```python
from build123d import *
from build123d.topology import SkipClean

# Parameters (mm, degrees)
ESBO_O1_R                  = 0.75
ESBO_O1_R_2                = 1.5
RESSALTO_EXTRUS_O1_DEPTH   = 2
ESBO_O3_R                  = 3.75
ESBO_O3_R_2                = 2.5
RESSALTO_EXTRUS_O2_DEPTH   = 1.5
RESSALTO_EXTRUS_O3_DEPTH   = 1.5
CORTE_EXTRUS_O1_DEPTH      = 19.95718861
CORTE_EXTRUS_O1_DEPTH_BACK = 19.95718861
RESSALTO_EXTRUS_O4_START   = 2
ESBO_O7_R                  = 3.75
ESBO_O7_R_2                = 1.5
RESSALTO_EXTRUS_O4_DEPTH   = 2
ESBO_O8_R                  = 2.5
CORTE_EXTRUS_O2_DEPTH      = 3
RESSALTO_EXTRUS_O5_START   = 3
RESSALTO_EXTRUS_O5_DEPTH   = 3


with BuildPart() as part:
    # Esboço1 → Ressalto-extrusão1 (new body)
    with BuildSketch(Plane(origin=(0, 0, 0), x_dir=(1, 0, 0), z_dir=(0, 1, 0))):
        with BuildLine():
            Line((0.297619048, 3.738171064), (15.948412698, 2.492114043))
            ThreePointArc((15.948412698, 2.492114043), (18.25, 0), (15.948412698, -2.492114043))
            Line((15.948412698, -2.492114043), (0.297619048, -3.738171064))
            ThreePointArc((0.297619048, -3.738171064), (-3.75, 0), (0.297619048, 3.738171064))
        make_face()
        with Locations(Location((15.75, 0, 0), (0, 0, 270))):
            Circle(ESBO_O1_R, mode=Mode.SUBTRACT)
        with Locations(Location((0, 0, 0), (0, 0, 270))):
            Circle(ESBO_O1_R_2, mode=Mode.SUBTRACT)
        with Locations(Location((13.25, 0, 0), (0, 0, 270))):
            Circle(ESBO_O1_R, mode=Mode.SUBTRACT)
        with Locations(Location((10.75, 0, 0), (0, 0, 270))):
            Circle(ESBO_O1_R, mode=Mode.SUBTRACT)
        with Locations(Location((8.25, 0, 0), (0, 0, 270))):
            Circle(ESBO_O1_R, mode=Mode.SUBTRACT)
        with Locations(Location((5.75, 0, 0), (0, 0, 270))):
            Circle(ESBO_O1_R, mode=Mode.SUBTRACT)
    extrude(amount=RESSALTO_EXTRUS_O1_DEPTH)

    # Esboço3 → Ressalto-extrusão2 (add)
    with SkipClean():  # the faces are left unmerged after this step: merging them gives an invalid solid
        with BuildSketch(Plane(origin=(0, 2, 0), x_dir=(1, 0, 0), z_dir=(0, 1, 0))):
            with Locations(Location((0, 0, 0), (0, 0, 85.447928579))):
                Circle(ESBO_O3_R)
            with Locations(Location((0, 0, 0), (0, 0, 270))):
                Circle(ESBO_O3_R_2, mode=Mode.SUBTRACT)
        extrude(amount=RESSALTO_EXTRUS_O2_DEPTH)

    # Esboço5 → Ressalto-extrusão3 (add)
    with SkipClean():  # the faces are left unmerged after this step: merging them gives an invalid solid
        with BuildSketch(Plane(origin=(0, 2, 0), x_dir=(1, 0, 0), z_dir=(0, 1, 0))):
            with BuildLine():
                Line((5, 2.360620906), (5, 3.36378527))
                Line((5, 3.36378527), (0.297619048, 3.738171064))
                ThreePointArc((0.297619048, 3.738171064), (1.642055332, 3.37137276), (2.759721595, 2.538983403))
                Line((2.759721595, 2.538983403), (5, 2.360620906))
            make_face()
            with BuildLine():
                Line((5, 0.5), (3.716517187, 0.5))
                ThreePointArc((3.716517187, 0.5), (3.75, 0), (3.716517187, -0.5))
                Line((3.716517187, -0.5), (5, -0.5))
                Line((5, -0.5), (5, 0.5))
            make_face()
            with BuildLine():
                Line((5, -2.360620906), (2.759721595, -2.538983403))
                ThreePointArc((2.759721595, -2.538983403), (1.642055332, -3.37137276), (0.297619048, -3.738171064))
                Line((0.297619048, -3.738171064), (5, -3.36378527))
                Line((5, -3.36378527), (5, -2.360620906))
            make_face()
        extrude(amount=RESSALTO_EXTRUS_O3_DEPTH)

    # Esboço6 → Corte-extrusão1 (cut, two sides: drawn at the far end of the back side and taken through both)
    with SkipClean():  # the faces are left unmerged after this step: merging them gives an invalid solid
        with BuildSketch(Plane.XY.offset(-CORTE_EXTRUS_O1_DEPTH_BACK)):
            Polygon((3.716517187, 3.5), (5, 2), (5, 3.5), align=None)
        extrude(amount=CORTE_EXTRUS_O1_DEPTH + CORTE_EXTRUS_O1_DEPTH_BACK, mode=Mode.SUBTRACT)

    # Esboço7 → Ressalto-extrusão4 (add)
    with SkipClean():  # the faces are left unmerged after this step: merging them gives an invalid solid
        with BuildSketch(Plane.XZ.offset(RESSALTO_EXTRUS_O4_START)):
            with Locations(Location((0, 0, 0), (0, 0, 270))):
                Circle(ESBO_O7_R)
            with Locations(Location((0, 0, 0), (0, 0, 270))):
                Circle(ESBO_O7_R_2, mode=Mode.SUBTRACT)
        extrude(amount=-RESSALTO_EXTRUS_O4_DEPTH)

    # Esboço8 → Corte-extrusão2 (cut)
    with SkipClean():  # the faces are left unmerged after this step: merging them gives an invalid solid
        with BuildSketch(Plane.XZ.offset(2)):
            with Locations(Location((0, 0, 0), (0, 0, 90))):
                Circle(ESBO_O8_R)
        extrude(amount=-CORTE_EXTRUS_O2_DEPTH, mode=Mode.SUBTRACT)

    # Esboço9 → Ressalto-extrusão5 (add)
    with SkipClean():  # the faces are left unmerged after this step: merging them gives an invalid solid
        with BuildSketch(Plane.XZ.offset(-1).offset(RESSALTO_EXTRUS_O5_START)):
            with BuildLine():
                Line((-0.3, 2.481934729), (0, 2.181934729))
                Line((0, 2.181934729), (0.3, 2.481934729))
                ThreePointArc((0.3, 2.481934729), (0, 2.5), (-0.3, 2.481934729))
            make_face()
            with BuildLine():
                Line((0.444891262, 2.460095885), (0.643136552, 2.084997491))
                Line((0.643136552, 2.084997491), (1.018234946, 2.283242781))
                ThreePointArc((1.018234946, 2.283242781), (0.736887936, 2.388932014), (0.444891262, 2.460095885))
            make_face()
            with BuildLine():
                Line((1.150251983, 2.219666726), (1.229127598, 1.802799076))
                Line((1.229127598, 1.802799076), (1.645995248, 1.881674691))
                ThreePointArc((1.645995248, 1.881674691), (1.408300145, 2.065596936), (1.150251983, 2.219666726))
            make_face()
            with BuildLine():
                Line((1.753407768, 1.782010437), (1.705905264, 1.360414052))
                Line((1.705905264, 1.360414052), (2.127501649, 1.312911548))
                ThreePointArc((2.127501649, 1.312911548), (1.954578706, 1.558724505), (1.753407768, 1.782010437))
            make_face()
            with BuildLine():
                Line((2.200765578, 1.186014701), (2.031105761, 0.797150269))
                Line((2.031105761, 0.797150269), (2.419970193, 0.627490452))
                ThreePointArc((2.419970193, 0.627490452), (2.327184372, 0.913352561), (2.200765578, 1.186014701))
            make_face()
            with BuildLine():
                Line((2.452575708, 0.484636354), (2.175833597, 0.163056187))
                Line((2.175833597, 0.163056187), (2.497413764, -0.113685925))
                ThreePointArc((2.497413764, -0.113685925), (2.493009493, 0.186825234), (2.452575708, 0.484636354))
            make_face()
            with BuildLine():
                Line((2.486463724, -0.25980406), (2.12722907, -0.485526154))
                Line((2.12722907, -0.485526154), (2.352951164, -0.844760808))
                ThreePointArc((2.352951164, -0.844760808), (2.43731978, -0.556302335), (2.486463724, -0.25980406))
            make_face()
            with BuildLine():
                Line((2.299418526, -0.981159743), (1.889610905, -1.090967365))
                Line((1.889610905, -1.090967365), (1.999418526, -1.500774986))
                ThreePointArc((1.999418526, -1.500774986), (2.165063509, -1.25), (2.299418526, -0.981159743))
            make_face()
            with BuildLine():
                Line((1.908059901, -1.615335078), (1.484092518, -1.599471337))
                Line((1.484092518, -1.599471337), (1.468228778, -2.02343872))
                ThreePointArc((1.468228778, -2.02343872), (1.700431844, -1.83262968), (1.908059901, -1.615335078))
            make_face()
            with BuildLine():
                Line((1.347161781, -2.105980801), (0.946705999, -1.965855263))
                Line((0.946705999, -1.965855263), (0.80658046, -2.366311045))
                ThreePointArc((0.80658046, -2.366311045), (1.084709348, -2.25242217), (1.347161781, -2.105980801))
            make_face()
            with BuildLine():
                Line((0.666562424, -2.409500889), (0.325200497, -2.157564321))
                Line((0.325200497, -2.157564321), (0.073263929, -2.498926249))
                ThreePointArc((0.073263929, -2.498926249), (0.372605665, -2.472077066), (0.666562424, -2.409500889))
            make_face()
            with BuildLine():
                Line((-0.073263929, -2.498926249), (-0.325200497, -2.157564321))
                Line((-0.325200497, -2.157564321), (-0.666562424, -2.409500889))
                ThreePointArc((-0.666562424, -2.409500889), (-0.372605665, -2.472077066), (-0.073263929, -2.498926249))
            make_face()
            with BuildLine():
                Line((-0.80658046, -2.366311045), (-0.946705999, -1.965855263))
                Line((-0.946705999, -1.965855263), (-1.347161781, -2.105980801))
                ThreePointArc((-1.347161781, -2.105980801), (-1.084709348, -2.25242217), (-0.80658046, -2.366311045))
            make_face()
            with BuildLine():
                Line((-1.468228778, -2.02343872), (-1.484092518, -1.599471337))
                Line((-1.484092518, -1.599471337), (-1.908059901, -1.615335078))
                ThreePointArc((-1.908059901, -1.615335078), (-1.700431844, -1.83262968), (-1.468228778, -2.02343872))
            make_face()
            with BuildLine():
                Line((-1.999418526, -1.500774986), (-1.889610905, -1.090967365))
                Line((-1.889610905, -1.090967365), (-2.299418526, -0.981159743))
                ThreePointArc((-2.299418526, -0.981159743), (-2.165063509, -1.25), (-1.999418526, -1.500774986))
            make_face()
            with BuildLine():
                Line((-2.352951164, -0.844760808), (-2.12722907, -0.485526154))
                Line((-2.12722907, -0.485526154), (-2.486463724, -0.25980406))
                ThreePointArc((-2.486463724, -0.25980406), (-2.43731978, -0.556302335), (-2.352951164, -0.844760808))
            make_face()
            with BuildLine():
                Line((-2.497413764, -0.113685925), (-2.175833597, 0.163056187))
                Line((-2.175833597, 0.163056187), (-2.452575708, 0.484636354))
                ThreePointArc((-2.452575708, 0.484636354), (-2.493009493, 0.186825234), (-2.497413764, -0.113685925))
            make_face()
            with BuildLine():
                Line((-2.419970193, 0.627490452), (-2.031105761, 0.797150269))
                Line((-2.031105761, 0.797150269), (-2.200765578, 1.186014701))
                ThreePointArc((-2.200765578, 1.186014701), (-2.327184372, 0.913352561), (-2.419970193, 0.627490452))
            make_face()
            with BuildLine():
                Line((-2.127501649, 1.312911548), (-1.705905264, 1.360414052))
                Line((-1.705905264, 1.360414052), (-1.753407768, 1.782010437))
                ThreePointArc((-1.753407768, 1.782010437), (-1.954578706, 1.558724505), (-2.127501649, 1.312911548))
            make_face()
            with BuildLine():
                Line((-1.645995248, 1.881674691), (-1.229127598, 1.802799076))
                Line((-1.229127598, 1.802799076), (-1.150251983, 2.219666726))
                ThreePointArc((-1.150251983, 2.219666726), (-1.408300145, 2.065596936), (-1.645995248, 1.881674691))
            make_face()
            with BuildLine():
                Line((-1.018234946, 2.283242781), (-0.643136552, 2.084997491))
                Line((-0.643136552, 2.084997491), (-0.444891262, 2.460095885))
                ThreePointArc((-0.444891262, 2.460095885), (-0.736887936, 2.388932014), (-1.018234946, 2.283242781))
            make_face()
        extrude(amount=-RESSALTO_EXTRUS_O5_DEPTH)


solid = part.part
```
Check sheet for the modelled part. Datum: model origin and axes. Units: mm. A direction names the side the tool comes from. Give positions to 0.01 mm unless a question says otherwise; leave off trailing zeros. Write each loop counter-clockwise with the first axis right and the second up, starting at its lowest first coordinate (ties: lowest second). Pieces come first, ordered by that corner, then holes. Notation, with made-up numbers: (46, 39.25) - (77, 39.25) arc R24 cw to (77, 69.25) - close; hole circle Ø2 at (-31, -6.5). An arc over 180 degrees is marked (long way). Answer as a JSON object with one key per item and string values. Group by question number.
1) Release check for a two-part mould opening along Z. For faces 4 (the face through (18.25, 0.99, -0.05)), 5 (the face through (5.975, 0.986, 0.715)), 6 (the face through (2, -2, -2)) record: pulls with the +Z half, pulls with the -Z half, needs draft (parallel to the pull), parting line crosses it, or undercut.
2) Sectioned sample at C-C (x = 15.75). Record the cut outline in (y, z).
3) Sectioned sample at B-B (x = 5.75). Record the cut outline in (y, z).
4) Depth check by flat-ended pin: P1, Ø0.9, axis at x = 8.25, z = 0, coming from the -Y side; P2, Ø1.7, axis at x = 15.75, z = 0, coming from the +Y side; P3, Ø1, axis at y = 1, z = -3, coming from the -X side; P4, Ø2, axis at x = 11.5, z = -1, coming from the -Y side. Enter the tip coordinate at first touch or a pass-through.
5) Thickness scan on probe 1 along Z at (x, y) = (3, 2.2); probe 2 along Z at (x, y) = (4, 2.95); probe 3 along Y at (x, z) = (7, -1.5). Record the ranges inside material, lowest first. Write a range as from..to.
6) Sectioned sample at A-A (y = 1.6). Record the cut outline in (x, z), then the cut area to 3 significant figures.
7) Sectioned sample at D-D (x = 12.25). Record the cut outline in (y, z), then the cut area to 3 significant figures.
8) Access from +Z, -Z, +X, -X, +Y, -Y to the whole of each face (thin tool, end or side, straight path). Record for faces 1 (the face through (4.1, 2.4, -0.5)), 2 (the face through (0, 2, 2)), 3 (the face through (11.382, 0.986, 0.403)).
Geometry results:
{
 "1": {"face 4": "parting line crosses it", "face 5": "undercut", "face 6": "needs draft"},
 "2": {"outline": "(0, -2.51) - (2, -2.51) - (2, -0.75) - (0, -0.75) - close; (0, 0.75) - (2, 0.75) - (2, 2.51) - (0, 2.51) - close"},
 "3": {"outline": "(0, -3.3) - (2, -3.3) - (2, -0.75) - (0, -0.75) - close; (0, 0.75) - (2, 0.75) - (2, 3.3) - (0, 3.3) - close"},
 "4": {"P1": "passes through", "P2": "stops at y = 2", "P3": "stops at x = -2.8", "P4": "stops at y = 0"},
 "5": {"probe 1": "z = -3.52..-2.52, -2.25..2.25, 2.52..3.52", "probe 2": "z = -3.44..-2.44, -0.5..0.5, 2.44..3.44", "probe 3": "y = 0..2"},
 "6": {"outline": "(0.3, -3.74) - (15.95, -2.49) arc R2.5 ccw to (15.95, 2.49) - (0.3, 3.74) arc R3.75 ccw (long way) to start; hole circle Ø3 at (0, 0); hole circle Ø1.5 at (5.75, 0); hole circle Ø1.5 at (8.25, 0); hole circle Ø1.5 at (10.75, 0); hole circle Ø1.5 at (13.25, 0); hole circle Ø1.5 at (15.75, 0)", "area": "115 mm^2"},
 "7": {"outline": "(0, -2.79) - (2, -2.79) - (2, 2.79) - (0, 2.79) - close", "area": "11.1 mm^2"},
 "8": {"face 1": "+X, +Y", "face 2": "+Y", "face 3": "+Y, -Y"}
}
